from build123d import *

# Parameters (mm, degrees)
AUFSATZ_LINEAR_AUSTRAGEN1_DEPTH            = 30
DURCHGANGSLOCH_F_R_M51_D                   = 5.3
DURCHGANGSLOCH_F_R_M43_REACH               = 68.321
DURCHGANGSLOCH_F_R_M43_BORE_R              = 2.15
DURCHGANGSLOCH_F_R_M41_D                   = 4.3
DURCHGANGSLOCH_F_R_M41_CSINK_D             = 4.35
DURCHGANGSLOCH_F_R_M41_CSINK_ANGLE         = 90
SKIZZE21_W                                 = 40
SKIZZE21_H                                 = 20
SCHNITT_LINEAR_AUSTRAGEN5_DEPTH            = 22
SKIZZE22_R                                 = 6.05
SCHNITT_LINEAR_AUSTRAGEN6_DEPTH            = 4.5
F_6_2_6_2_DURCHMESSER_BOHRUNG1_D           = 6.2
F_6_2_6_2_DURCHMESSER_BOHRUNG1_CSINK_D     = 6.25
F_6_2_6_2_DURCHMESSER_BOHRUNG1_CSINK_ANGLE = 90
SKIZZE25_R                                 = 6.05
SCHNITT_LINEAR_AUSTRAGEN7_DEPTH            = 4
DURCHGANGSLOCH_F_R_M42_D                   = 4.3
DURCHGANGSLOCH_F_R_M42_DEPTH               = 9
DURCHGANGSLOCH_F_R_M42_CSINK_D             = 4.35
DURCHGANGSLOCH_F_R_M42_CSINK_ANGLE         = 90
DURCHGANGSLOCH_F_R_M42_TIP                 = 1.291850331
SKIZZE30_W                                 = 36
SKIZZE30_H                                 = 2
SCHNITT_LINEAR_AUSTRAGEN8_DEPTH            = 23


with BuildPart() as part:
    # Skizze1 → Aufsatz-Linear austragen1 (new body)
    with BuildSketch(Plane.XY):
        Polygon((26.428839574, -31.372693626), (-43.571160426, -31.372693626), (-43.571160426, 8.627306374), (-23.571160426, 8.627306374), (-13.068047352, -6.372693626), (-4.074273499, -6.372693626), (6.428839574, 8.627306374), (26.428839574, 8.627306374), align=None)
    extrude(amount=AUFSATZ_LINEAR_AUSTRAGEN1_DEPTH)

    # Durchgangsloch für M51 (through all)
    with Locations(Plane.XY.offset(30)):
        with Locations((-36.571160426, -22.872693626), (19.428839574, -22.872693626)):
            Hole(DURCHGANGSLOCH_F_R_M51_D / 2)

    # Durchgangsloch für M43 bore → Durchgangsloch für M43 (cut, up to next)
    with BuildSketch(Plane(origin=(0, -31.372693626, 0), x_dir=(-1, 0, 0), z_dir=(0, -1, 0)), mode=Mode.PRIVATE) as durchgangsloch_f_r_m43_sk1:
        with Locations((36.571160426, -15)):
            Circle(DURCHGANGSLOCH_F_R_M43_BORE_R)
    durchgangsloch_f_r_m43_tool1 = extrude(durchgangsloch_f_r_m43_sk1.sketch, amount=-DURCHGANGSLOCH_F_R_M43_REACH, mode=Mode.PRIVATE) & part.part
    # Durchgangsloch für M43 bore → Durchgangsloch für M43 (cut, up to next)
    with BuildSketch(Plane(origin=(0, -31.372693626, 0), x_dir=(-1, 0, 0), z_dir=(0, -1, 0)), mode=Mode.PRIVATE) as durchgangsloch_f_r_m43_sk2:
        with Locations((-19.428839574, -15)):
            Circle(DURCHGANGSLOCH_F_R_M43_BORE_R)
    durchgangsloch_f_r_m43_tool2 = extrude(durchgangsloch_f_r_m43_sk2.sketch, amount=-DURCHGANGSLOCH_F_R_M43_REACH, mode=Mode.PRIVATE) & part.part
    add(durchgangsloch_f_r_m43_tool1.solids().sort_by_distance((-36.57116, -31.372694, 15))[0], mode=Mode.SUBTRACT)
    add(durchgangsloch_f_r_m43_tool2.solids().sort_by_distance((19.42884, -31.372694, 15))[0], mode=Mode.SUBTRACT)

    # Durchgangsloch für M41 (through all)
    with Locations(Plane(origin=(0, 0, 0), x_dir=(-1, 0, 0), z_dir=(0, 0, -1))):
        with Locations((-22.428839574, 4.627306374), (-22.428839574, -16.372693626), (39.571160426, -16.372693626), (39.571160426, 4.627306374)):
            CounterSinkHole(DURCHGANGSLOCH_F_R_M41_D / 2, DURCHGANGSLOCH_F_R_M41_CSINK_D / 2, counter_sink_angle=DURCHGANGSLOCH_F_R_M41_CSINK_ANGLE)

    # Skizze21 → Schnitt-Linear austragen5 (cut)
    with BuildSketch(Plane.XZ.offset(31.372693626)):
        with Locations((-8.571160426, 16)):
            Rectangle(SKIZZE21_W, SKIZZE21_H)
    extrude(amount=-SCHNITT_LINEAR_AUSTRAGEN5_DEPTH, mode=Mode.SUBTRACT)

    # Skizze22 → Schnitt-Linear austragen6 (cut)
    with BuildSketch(Plane(origin=(0, 0, 0), x_dir=(-1, 0, 0), z_dir=(0, 0, -1))):
        with Locations((8.571160426, -22.872693626)):
            Circle(SKIZZE22_R)
    extrude(amount=-SCHNITT_LINEAR_AUSTRAGEN6_DEPTH, mode=Mode.SUBTRACT)

    # Ø6.2 (6.2) Durchmesser Bohrung1 (through all)
    with Locations(Plane(origin=(0, 0, 4.5), x_dir=(-1, 0, 0), z_dir=(0, 0, -1))):
        with Locations((8.571160426, -22.872693626)):
            CounterSinkHole(F_6_2_6_2_DURCHMESSER_BOHRUNG1_D / 2, F_6_2_6_2_DURCHMESSER_BOHRUNG1_CSINK_D / 2, counter_sink_angle=F_6_2_6_2_DURCHMESSER_BOHRUNG1_CSINK_ANGLE)

    # Skizze25 → Schnitt-Linear austragen7 (cut)
    with BuildSketch(Plane.XY.offset(30)):
        with Locations(Location((-8.571160426, -22.872693626, 0), (0, 0, 180))):
            Circle(SKIZZE25_R)
    extrude(amount=-SCHNITT_LINEAR_AUSTRAGEN7_DEPTH, mode=Mode.SUBTRACT)

    # Durchgangsloch für M42
    with Locations(Plane(origin=(0, 8.627306374, 0), x_dir=(1, 0, 0), z_dir=(0, 1, 0))):
        with Locations((-33.571160426, -15), (16.428839574, -15)):
            CounterSinkHole(DURCHGANGSLOCH_F_R_M42_D / 2, DURCHGANGSLOCH_F_R_M42_CSINK_D / 2, depth=DURCHGANGSLOCH_F_R_M42_DEPTH, counter_sink_angle=DURCHGANGSLOCH_F_R_M42_CSINK_ANGLE)
            with Locations((0, 0, -(DURCHGANGSLOCH_F_R_M42_DEPTH + DURCHGANGSLOCH_F_R_M42_TIP / 2))):  # 118° drill point
                Cone(0, DURCHGANGSLOCH_F_R_M42_D / 2, DURCHGANGSLOCH_F_R_M42_TIP, mode=Mode.SUBTRACT)

    # Skizze30 → Schnitt-Linear austragen8 (cut)
    with BuildSketch(Plane(origin=(0, 8.627306374, 0), x_dir=(1, 0, 0), z_dir=(0, 1, 0))):
        with Locations((-8.571160426, -4)):
            Rectangle(SKIZZE30_W, SKIZZE30_H)
    extrude(amount=-SCHNITT_LINEAR_AUSTRAGEN8_DEPTH, mode=Mode.SUBTRACT)


solid = part.part
Design review of the part built by this model. Coordinates are the model's own, in mm. A direction names the side the tool comes from. Round coordinates to 2 decimals unless told otherwise and drop trailing zeros. Write each loop counter-clockwise with the first axis right and the second up, starting at its lowest first coordinate (ties: lowest second). Pieces come first, ordered by that corner, then holes. Notation, with made-up numbers: (67, 14.5) - (114, 14.5) arc R23 ccw to (114, 33.5) - close; hole circle Ø1 at (-19.5, -22.75). An arc over 180 degrees is marked (long way). Return JSON: item names as keys, results as strings. Group by question number.
Item 1: We need section C-C on x = -10.5. Give the number of separate pieces and of enclosed holes in the cut face, and give its area (3 significant figures).
Item 2: We need section B-B on y = -12.5. Write out the cut boundary in (x, z).
Item 3: The part is to be moulded in two halves that separate along X. For faces 5 (the face through (-36.226, -20.245, 14.79)), 6 (the face through (-36, 8.627, 15)), 7 (the face through (26.429, -11, 15)), 8 (the face through (1.1, 1.02, 1.48)), say which applies: pulls with the +X half, pulls with the -X half, needs draft (parallel to the pull), parting line crosses it, or undercut.
Item 4: We need section A-A on z = 9.5. Write out the cut boundary in (x, y).
Item 5: Insertion check: P1, Ø7, axis at x = -9.5, y = -5, coming from the -Z side; P2, Ø3.5, axis at x = -8.57, y = -22.87, coming from the +Z side; P3, Ø1.5, axis at x = -19.5, z = 9.5, coming from the +Y side; P4, Ø4, axis at x = -33.57, z = 15, coming from the +Y side. Each pin has a flat end and moves straight along its axis. Give the tip position at first contact, or say it passes through.
Item 6: For probe 1 along Z at (x, y) = (-10, -12); probe 2 along X at (y, z) = (-26.5, 15); probe 3 along Z at (x, y) = (-15, -7), list the stretches that pass through material, from the lowest coordinate up. Write a range as [from, to].
Item 7: Machinability: for faces 1 (the face through (-18.39, 1.23, 1.48)), 2 (the face through (18, -20.64, 14.79)), 3 (the face through (-9, -18, 6)), 4 (the face through (9.429, -3, 4)), which of the approach directions +Z, -Z, +X, -X, +Y, -Y give a long, thin tool a straight path to every point of the face, cutting with its end or side? Answer none if there is none.
Model answer:
{
 "1": {"separate pieces": "3", "enclosed holes": "0", "area": "189 mm²"},
 "2": {"outline": "(-43.57, 0) - (26.43, 0) - (26.43, 30) - (-43.57, 30) - close; hole (-28.57, 6) - (11.43, 6) - (11.43, 26) - (-28.57, 26) - close; hole (-26.57, 3) - (9.43, 3) - (9.43, 5) - (-26.57, 5) - close"},
 "3": {"face 5": "undercut", "face 6": "needs draft", "face 7": "pulls with the +X half", "face 8": "undercut"},
 "4": {"outline": "(-43.57, -31.37) - (-28.57, -31.37) - (-28.57, -9.37) - (11.43, -9.37) - (11.43, -31.37) - (26.43, -31.37) - (26.43, 8.63) - (6.43, 8.63) - (-4.07, -6.37) - (-13.07, -6.37) - (-23.57, 8.63) - (-43.57, 8.63) - close; hole circle Ø4.3 at (-39.57, -16.37); hole circle Ø4.3 at (-39.57, 4.63); hole circle Ø5.3 at (-36.57, -22.87); hole circle Ø5.3 at (19.43, -22.87); hole circle Ø4.3 at (22.43, -16.37); hole circle Ø4.3 at (22.43, 4.63)"},
 "5": {"P1": "stops at z = 0", "P2": "passes through", "P3": "stops at y = 3.88", "P4": "stops at y = -0.46"},
 "6": {"probe 1": "z = [0, 3], [5, 6], [26, 30]", "probe 2": "x = [-43.57, -38.72], [-34.42, -28.57], [11.43, 17.28], [21.58, 26.43]", "probe 3": "z = [0, 3], [5, 30]"},
 "7": {"face 1": "+Z, -Z, +Y", "face 2": "+Z, -Z", "face 3": "-Y", "face 4": "+Y"}
}
